```python
from build123d import *

# Parameters (mm, degrees)
SKETCH1_R           = 9.5
SKETCH1_R_2         = 1.5
BOSS_EXTRUDE1_DEPTH = 2.25


with BuildPart() as part:
    # Sketch1 → Boss-Extrude1 (new body)
    with BuildSketch(Plane(origin=(0, 0, 0), x_dir=(1, 0, 0), z_dir=(0, 1, 0))):
        Circle(SKETCH1_R)
        with Locations((-2.952501305, 1.996568505)):
            Circle(SKETCH1_R_2, mode=Mode.SUBTRACT)
        with BuildLine():
            Line((1.210041518, 3.303413345), (2.178074733, 3.303413345))
            add(Edge.make_bspline(
                [(2.178074733, 3.303413345), (2.444856065, 0.149541279), (-2.085629529, -1.114991667), (-3.758110102, -3.954281272), (-3.896333689, -5.820299703)],
                knots=[0, 0, 0, 0, 0.63008416, 1, 1, 1, 1], degree=3))
            Line((-3.896333689, -5.820299703), (-1.896333689, -5.820299703))
            add(Edge.make_bspline(
                [(4.186743653, 3.303413345), (4.162331661, 1.716633845), (3.916646292, 0.656016278), (2.663767731, -1.102040856), (1.822435365, -1.678254748), (0.735292504, -2.593233031), (-1.88135337, -3.72928874), (-1.896333689, -5.820299703)],
                knots=[0, 0, 0, 0, 0.433164655, 0.505148227, 0.695981554, 0.747852148, 1, 1, 1, 1], degree=3))
            Line((4.186743653, 3.303413345), (5.203178529, 3.303413345))
            Line((5.203178529, 3.303413345), (3.206610024, 6.304316311))
            Line((3.206610024, 6.304316311), (1.210041518, 3.303413345))
        make_face(mode=Mode.SUBTRACT)
    extrude(amount=BOSS_EXTRUDE1_DEPTH)


solid = part.part
```
Check sheet for the modelled part. Datum: model origin and axes. Units: mm. A direction names the side the tool comes from. Coordinates: 2 decimals unless noted, no trailing zeros. Loops run counter-clockwise (first coordinate to the right, second up) from the corner with the lowest first, then second, coordinate; pieces in that order, holes last.
1) Sectioned sample at C-C (x = -5.25). Record the boundary of the cut face in (y, z).
2) Sectioned sample at B-B (x = -3). Count the separate pieces of the cut face and the enclosed holes in it, and give its area (3 significant figures).
3) Access from +Z, -Z, +X, -X, +Y, -Y to the whole of each face (thin tool, end or side, straight path). Record for faces 5 (the face through (-3, 1, 5.82)), 6 (the face through (0, 0, 0)).
4) Material ranges on probe 1 along X at (y, z) = (0.6, -2); probe 2 along X at (y, z) = (1.45, -0.75); probe 3 along Z at (x, y) = (4.25, 2), recorded low to high.
5) Sectioned sample at A-A (z = -4.5). Record the boundary of the cut face in (x, y).
6) Release check for a two-part mould opening along X. For faces 1 (the face through (-4.06, 1.11, -3.01)), 2 (the face through (4.22, 1.11, -4.78)), 3 (the face through (0, 2.25, 0)), 4 (the face through (4.38, 1.11, 8.43)) record: released by +X, released by -X, zero draft, split by the parting line, or undercut.
Check sheet entries:
1. outline: (0, -7.92) - (2.25, -7.92) - (2.25, 7.92) - (0, 7.92) - close
2. separate pieces: 3
2. enclosed holes: 0
2. area: 27.4 mm2
3. face 5: +Y, -Y
3. face 6: +Z, -Z, +X, -X, -Y
4. probe 1: x = -9.29 to -4.45, -1.45 to 2.09, 4.1 to 9.29
4. probe 2: x = -9.47 to -3.79, -2.12 to 1.51, 3.79 to 9.47
4. probe 3: z = -8.5 to -4.74, -3.3 to 8.5
5. outline: (-8.37, 0) - (2.01, 0) - (2.01, 2.25) - (-8.37, 2.25) - close; (4.41, 0) - (8.37, 0) - (8.37, 2.25) - (4.41, 2.25) - close
6. face 1: undercut
6. face 2: undercut
6. face 3: zero draft
6. face 4: split by the parting line
